Check sheet for the modelled part. Datum: model origin and axes. Units: mm. Face numbers are marked on the shaded views. A direction names the side the tool comes from. Give positions to 0.01 mm unless a question says otherwise; leave off trailing zeros. Loops run counter-clockwise (first coordinate to the right, second up) from the corner with the lowest first, then second, coordinate; pieces in that order, holes last. Notation, with made-up numbers: M 49,49.25 L 70,49.25 A28 cw 70,76.25 Z; hole C 11.25,-8 d3. An arc over 180 degrees is marked long. Use one line per item in the form item = value.
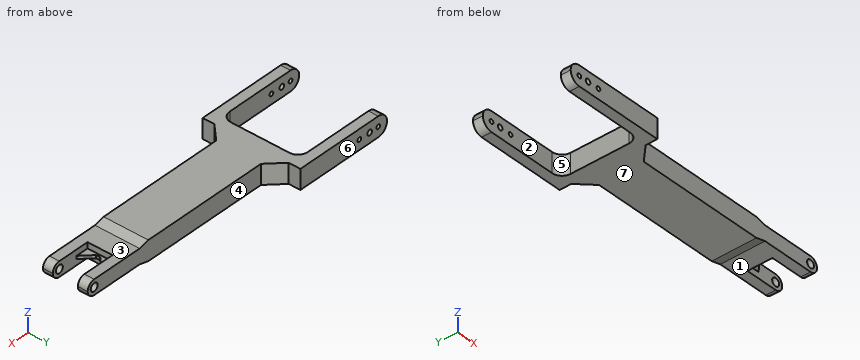
from build123d import *

# Parameters (mm, degrees)
SKETCH_2_W          = 165
SKETCH_2_H          = 45.3
EXTRUDE_1_DEPTH     = 10
EXTRUDE_2_DEPTH     = 7.5
CHAMFER_1_SIZE      = 20
CHAMFER_1_SIZE_2    = 5
CHAMFER_2_SIZE      = 5
CHAMFER_2_SIZE_2    = 20
EXTRUDE_3_DEPTH     = 1.5
CHAMFER_3_SIZE      = 3
CUT_EXTRUDE_1_DEPTH = 293.448286027
CUT_EXTRUDE_2_DEPTH = 285.483079462
CHAMFER_4_SIZE      = 15
FILLET_1_R          = 10


with BuildPart() as part:
    # 草图2 → 凸台-拉伸1 (new, symmetric)
    with BuildSketch(Plane.XY):
        with Locations((-92.5, 0)):
            Rectangle(SKETCH_2_W, SKETCH_2_H)
        Polygon((-275, 49.5), (-275, 39.5), (-185, 39.5), (-185, -39.5), (-275, -39.5), (-275, -49.5), (-175, -49.5), (-175, 49.5), align=None)
    extrude(amount=EXTRUDE_1_DEPTH, both=True)

    # 草图2<3> → 凸台-拉伸2 (add, symmetric)
    with BuildSketch(Plane.XY):
        Polygon((40, -22.65), (40, -12.65), (0, -12.65), (0, 12.65), (40, 12.65), (40, 22.65), (-10, 22.65), (-10, -22.65), align=None)
    extrude(amount=EXTRUDE_2_DEPTH, both=True)

    # 倒角1
    # the kernel refuses this chamfer: 20, 5 mm, written as the material it takes off along each edge
    with BuildSketch(Plane(origin=(-10, -74.592549995, 10), x_dir=(-0.9999563942249224, 0, 0.00933861064031752), z_dir=(0, 1, 0))) as chamfer_1_piece_1_section:
        Polygon((CHAMFER_1_SIZE * 0.999956394225, -CHAMFER_1_SIZE * 0.00933861064032), (-CHAMFER_1_SIZE_2 * 0.00933861064032, -CHAMFER_1_SIZE_2 * 0.999956394225), (0, 0), align=None)
    chamfer_1_piece_1 = extrude(amount=149.185099991, mode=Mode.PRIVATE)
    chamfer_1_piece_1 = split(chamfer_1_piece_1, bisect_by=Plane(origin=(-18.245866107, 0, 7.5), z_dir=(0, 0, 1)), keep=Keep.TOP, mode=Mode.PRIVATE)
    add(chamfer_1_piece_1, mode=Mode.SUBTRACT)

    # 倒角2
    # the kernel refuses this chamfer: 20, 5 mm, written as the material it takes off along each edge
    with BuildSketch(Plane(origin=(-10, -74.592549995, -10), x_dir=(0.14778356633657133, 0, 0.9890197255468893), z_dir=(0, 1, 0))) as chamfer_2_piece_1_section:
        Polygon((CHAMFER_2_SIZE * 0.989019725547, -CHAMFER_2_SIZE * 0.147783566337), (-CHAMFER_2_SIZE_2 * 0.147783566337, -CHAMFER_2_SIZE_2 * 0.989019725547), (0, 0), align=None)
    chamfer_2_piece_1 = extrude(amount=149.185099991, mode=Mode.PRIVATE)
    chamfer_2_piece_1 = split(chamfer_2_piece_1, bisect_by=Plane(origin=(-18.245866107, 0, -7.5), z_dir=(0, 0, -1)), keep=Keep.TOP, mode=Mode.PRIVATE)
    add(chamfer_2_piece_1, mode=Mode.SUBTRACT)

    # 草图2<5> → 凸台-拉伸3 (add, symmetric)
    with BuildSketch(Plane.XY):
        Polygon((12.65, 12.65), (0, 12.65), (0, 0), align=None)
        Polygon((12.65, -12.65), (0, 0), (0, -12.65), align=None)
    extrude(amount=EXTRUDE_3_DEPTH, both=True)

    # 倒角3
    chamfer_3_edges = [part.edges().sort_by_distance(p)[0] for p in [
        (0, 0, 0),
    ]]
    chamfer(chamfer_3_edges, length=CHAMFER_3_SIZE)

    # 草图3 → 切除-拉伸1 (cut, through all)
    with BuildSketch(Plane(origin=(0, 49.5, 0), x_dir=(1, 0, 0), z_dir=(0, 1, 0))):
        with BuildLine():
            ThreePointArc((-275, 0), (-272.071067812, 7.071067812), (-265, 10))
            Line((-265, 10), (-275, 10))
            Line((-275, 10), (-275, 0))
        make_face()
        with BuildLine():
            Line((-275, -10), (-265, -10))
            ThreePointArc((-265, -10), (-272.071067812, -7.071067812), (-275, 0))
            Line((-275, 0), (-275, -10))
        make_face()
        with BuildLine():
            ThreePointArc((-267.15, 0), (-265, -2.15), (-262.85, 0))
            Line((-262.85, 0), (-267.15, 0))
        make_face()
        with BuildLine():
            Line((-267.15, 0), (-262.85, 0))
            ThreePointArc((-262.85, 0), (-265, 2.15), (-267.15, 0))
        make_face()
        with BuildLine():
            ThreePointArc((-257.65, 0), (-255, -2.65), (-252.35, 0))
            Line((-252.35, 0), (-257.65, 0))
        make_face()
        with BuildLine():
            Line((-257.65, 0), (-252.35, 0))
            ThreePointArc((-252.35, 0), (-255, 2.65), (-257.65, 0))
        make_face()
        with BuildLine():
            ThreePointArc((-245.15, 0), (-243, -2.15), (-240.85, 0))
            Line((-240.85, 0), (-245.15, 0))
        make_face()
        with BuildLine():
            Line((-245.15, 0), (-240.85, 0))
            ThreePointArc((-240.85, 0), (-243, 2.15), (-245.15, 0))
        make_face()
    extrude(amount=-CUT_EXTRUDE_1_DEPTH, mode=Mode.SUBTRACT)

    # 草图4 → 切除-拉伸2 (cut, through all)
    with BuildSketch(Plane(origin=(0, 22.65, 0), x_dir=(1, 0, 0), z_dir=(0, 1, 0))):
        with BuildLine():
            ThreePointArc((28.5, 0), (32.5, -4), (36.5, 0))
            Line((36.5, 0), (28.5, 0))
        make_face()
        with BuildLine():
            Line((28.5, 0), (36.5, 0))
            ThreePointArc((36.5, 0), (32.5, 4), (28.5, 0))
        make_face()
        with BuildLine():
            ThreePointArc((32.5, 7.5), (37.803300859, 5.303300859), (40, 0))
            Line((40, 0), (40, 7.5))
            Line((40, 7.5), (32.5, 7.5))
        make_face()
        with BuildLine():
            Line((40, -7.5), (40, 0))
            ThreePointArc((40, 0), (37.80330088, -5.303300838), (32.500000061, -7.5))
            Line((32.500000061, -7.5), (40, -7.5))
        make_face()
    extrude(amount=-CUT_EXTRUDE_2_DEPTH, mode=Mode.SUBTRACT)

    # 倒角4
    chamfer_4_edges = [part.edges().sort_by_distance(p)[0] for p in [
        (-175, -22.65, 0),
        (-175, 22.65, 0),
    ]]
    chamfer(chamfer_4_edges, length=CHAMFER_4_SIZE)

    # 圆角1
    fillet_1_edges = [part.edges().sort_by_distance(p)[0] for p in [
        (-185, -39.5, 0),
        (-185, 39.5, 0),
    ]]
    fillet(fillet_1_edges, radius=FILLET_1_R)


solid = part.part
1) Depth check by flat-ended pin: pin 1 Ø1.8 at (y, z) = (-3.5, -4) entering from +X; pin 2 Ø1 at (x, z) = (-151, 4) entering from +Y; pin 3 Ø1 at (y, z) = (-17, 6) entering from -X. Enter the tip coordinate at first touch or a pass-through.
Evaluation:
pin_1 = 0
pin_2 = 22.65
pin_3 = -185
2) Section check B-B (x = -199). Record the cut outline in (y, z).
Evaluation:
outline = M -49.5,-10 L -39.5,-10 L -39.5,10 L -49.5,10 Z; M 39.5,-10 L 49.5,-10 L 49.5,10 L 39.5,10 Z
3) Section check C-C (y = 26). Record the cut outline in (x, z).
Evaluation:
outline = M -185,-10 L -163.35,-10 L -163.35,10 L -185,10 Z
4) Section check D-D (x = -99.5). Record the cut outline in (y, z), then the cut area to 3 significant figures.
Evaluation:
outline = M -22.65,-10 L 22.65,-10 L 22.65,10 L -22.65,10 Z
area = 906 mm^2
5) Section check A-A (x = -255). Record the cut outline in (y, z).
Evaluation:
outline = M -49.5,-10 L -39.5,-10 L -39.5,-2.65 L -49.5,-2.65 Z; M -49.5,2.65 L -39.5,2.65 L -39.5,10 L -49.5,10 Z; M 39.5,-10 L 49.5,-10 L 49.5,-2.65 L 39.5,-2.65 Z; M 39.5,2.65 L 49.5,2.65 L 49.5,10 L 39.5,10 Z
6) Set-up check for the marked faces 1, 2, 3 and 4: record each of +Z, -Z, +X, -X, +Y, -Y from which the full face is reachable in a straight line by a thin tool's end or side.
Evaluation:
face_1 = -Z, +X, +Y, -Y
face_2 = +Z, -Z, -X
face_3 = +Z, +X, +Y, -Y
face_4 = +Z, -Z, +X, +Y
7) Release check for a two-part mould opening along Y. For the marked faces 5, 6 and 7 record: pulls with the +Y half, pulls with the -Y half, needs draft (parallel to the pull), parting line crosses it, or undercut.
Evaluation:
face_5 = undercut
face_6 = pulls with the +Y half
face_7 = needs draft
8) Scan lines: line 1 (X direction, y = 40.5, z = 1.5); line 2 (Y direction, x = -254.5, z = 8.75); line 3 (X direction, y = -19.25, z = 0). Record each from-to range of solid material in increasing order.
Evaluation:
line_1 = -274.89 to -266.54, -263.46 to -257.18, -252.82 to -244.54, -241.46 to -175
line_2 = -49.5 to -39.5, 39.5 to 49.5
line_3 = -185 to 28.5, 36.5 to 40
